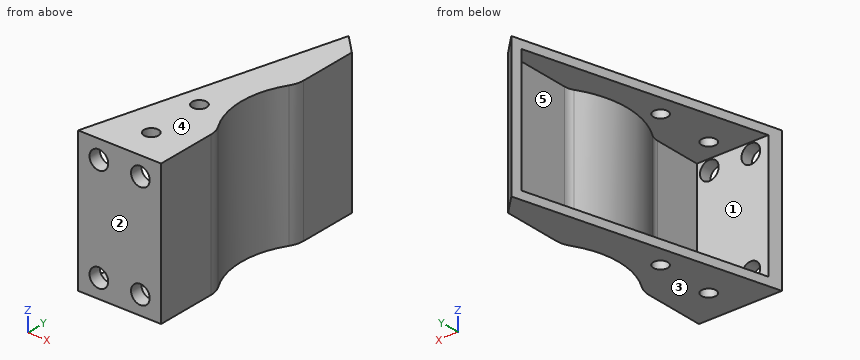
Autodesk Inventor part; units mm, degrees
ref_plane "YZ Plane" through (0, 0, 0) normal (1, 0, 0) x (0, 1, 0)
ref_plane "XZ Plane" through (0, 0, 0) normal (0, 1, 0) x (-1, 0, 0)
ref_plane "XY Plane" through (0, 0, 0) normal (0, 0, 1) x (1, 0, 0)
sketch "Sketch1" plane through (0, 0, 0) normal (0, 1, 0) x (-1, 0, 0)
  line L0 (0, 0) -> (-20, 0)
  line L1 (-20, 0) -> (-20, -34)
  line L2 (-20, -34) -> (0, -34)
  line L3 (0, -34) -> (0, 0)
  dimension "d0" = 34
  dimension "d1" = 20
extrude "Extrusion1" add sketch "Sketch1" along normal blind 60
chamfer "Chamfer1" distance 4.5 angle 45 1 edges at (20, 60, -17)
sketch "Sketch3" plane through (0, 0, 0) normal (0, 0, 1) x (1, 0, 0)
  line L0 (0, 60) -> (15.5, 60)
  line L1 (15.5, 60) -> (0, 0)
  line L2 (0, 0) -> (20, 0)
  line L3 (20, 0) -> (0, 0)
  line L4 (0, 0) -> (0, 60)
  line L5 (0, 60) -> (20, 60)
  line L6 (20, 60) -> (20, 0)
extrude "Extrusion2" cut sketch "Sketch3" against normal blind 60 contours L0 L1 L4
sketch "Sketch4" plane through (20, 0, -34) normal (0, 0, -1) x (-1, 0, 0)
  circle A0 centre (-16, 28) radius 19.8
  line L0 (0, 0) -> (0, 55.5)
  line L1 (20, 0) -> (0, 0)
  dimension "d9" = 39.6
  dimension "d14" = 16
  dimension "d15" = 28
extrude "Extrusion3" cut sketch "Sketch4" against normal blind 60
fillet "Fillet1" radius 6 2 edges at (20, 16.3364, -17) (20, 39.6636, -17)
shell "Shell1" thickness 2 removed faces 1 at (10.3333, 40, -22.6667)
sketch "Sketch5" plane through (0, 0, 0) normal (0, 0, 1) x (1, 0, 0)
  line L0 (0, 0) -> (20, 0)
  line L1 (20, 0) -> (-6.4586, 0)
  line L2 (-6.4586, 0) -> (-6.4586, 3)
  line L3 (-6.4586, 3) -> (20, 3)
  line L4 (20, 3) -> (20, 0)
  line L5 (0, 0) -> (0.775, 3)
  line L6 (15.5, 60) -> (0, 0)
  dimension "d16" = 3
extrude "Extrusion4" add sketch "Sketch5" against normal blind 34 contours L5 L3 L4 L0
sketch "Sketch6" plane through (0, 0, 0) normal (0, -1, 0) x (1, 0, 0)
  circle A0 centre (5, -4.5) radius 2.25
  line L0 (0, 0) -> (20, 0)
  line L1 (0, -34) -> (0, 0)
  circle A1 centre (15, -4.5) radius 2.25
  circle A2 centre (5, -29.5) radius 2.25
  circle A3 centre (15, -29.5) radius 2.25
  dimension "d19" = 4.5
  dimension "d20" = 4.5
  dimension "d21" = 5
  dimension "d24" = 10
  dimension "d27" = 25
extrude "Extrusion5" cut sketch "Sketch6" against normal blind 3
sketch "Sketch7" plane through (0, 0, 0) normal (0, 0, 1) x (1, 0, 0)
  circle A0 centre (11, 8) radius 1.75
  line L0 (0, 0) -> (20, 0)
  line L1 (20, 0) -> (20, 14.5226)
  line L2 (20, 0) -> (20, 15.3258)
  circle A1 centre (11, 22) radius 1.75
  dimension "d32" = 3.5
  dimension "d33" = 8
  dimension "d34" = 11
  dimension "d37" = 14
extrude "Extrusion6" cut sketch "Sketch7" against normal through all
properties part number "Gripper"
The model under review builds one solid part; all positions refer to its coordinate system, in mm. Face numbers are marked on the shaded views. A direction names the side the tool comes from. Give positions to 0.01 mm unless a question says otherwise; leave off trailing zeros. Write each loop counter-clockwise with the first axis right and the second up, starting at its lowest first coordinate (ties: lowest second). Pieces come first, ordered by that corner, then holes.
1. For P1, Ø2, axis at y = 38, z = -8, coming from the -X side; P2, Ø9, axis at y = 6.5, z = -10, coming from the -X side; P3, Ø12, axis at x = 4.5, z = -22, coming from the +Y side, all flat-tipped, find the tip position at first contact; note any pin that passes through.
2. Draft analysis for pull direction Y (two halves, no side actions). For the marked faces 1, 2 and 3, state which applies: +Y half, -Y half, draft (parallel to the pull), parting line (faces both ways), or undercut.
3. Add section A-A, the plane z = -29.5. Write out the cut boundary in (x, y) (3 decimals).
4. Add section C-C, the plane x = 5. Write out the cut boundary in (y, z).
5. Wall thickness on L1, parallel to Z at x = 5, y = 1.55; L2, parallel to Z at x = 4.5, y = 6.5; L3, parallel to X at y = 3.5, z = -25: over which ranges is each line inside the solid? List them lowest first.
6. Tool access review of the marked faces 4 and 5: name each direction out of +Z, -Z, +X, -X, +Y, -Y from which nothing blocks a thin tool from reaching the whole face with its end or side.
7. Add section D-D, the plane x = 10.5. Write out the cut boundary in (y, z).
8. Add section B-B, the plane y = 8. Write out the cut boundary in (x, z).
Worked answers:
1. P1: stops at x = 16.14
1. P2: stops at x = 0.52
1. P3: stops at y = 3
2. face 1: undercut
2. face 2: -Y half
2. face 3: draft
3. outline: (0, 0) - (2.75, 0) - (2.75, 3) - (0.775, 3) - close; (7.25, 0) - (12.75, 0) - (12.75, 3) - (7.25, 3) - close; (14.919, 57.752) - (18, 54.672) - (18, 41.477) arc R4 cw to (17.411, 39.388) arc R21.8 ccw to (17.411, 16.612) arc R4 cw to (18, 14.523) - (18, 3) - (17.25, 3) - (17.25, 0) - (20, 0) - (20, 14.523) arc R6 ccw to (19.116, 17.657) arc R19.8 cw to (19.116, 38.343) arc R6 ccw to (20, 41.477) - (20, 55.5) - (15.5, 60) - close
4. outline: (0, -34) - (19.35, -34) - (19.35, -32) - (3, -32) - (3, -31.75) - (0, -31.75) - close; (0, -27.25) - (3, -27.25) - (3, -6.75) - (0, -6.75) - close; (0, -2.25) - (3, -2.25) - (3, -2) - (19.35, -2) - (19.35, 0) - (0, 0) - close
5. L1: z = -34 to -31.75, -27.25 to -6.75, -2.25 to 0
5. L2: z = -34 to -32, -2 to 0
5. L3: x = 18 to 20
6. face 4: +Z, +X, -X, +Y, -Y
6. face 5: -X
7. outline: (0, -34) - (6.32, -34) - (6.32, -32) - (3, -32) - (3, -2) - (6.32, -2) - (6.32, 0) - (0, 0) - close; (9.68, -34) - (20.32, -34) - (20.32, -32) - (9.68, -32) - close; (9.68, -2) - (20.32, -2) - (20.32, 0) - (9.68, 0) - close; (23.68, -34) - (40.65, -34) - (40.65, -32) - (23.68, -32) - close; (23.68, -2) - (40.65, -2) - (40.65, 0) - (23.68, 0) - close
8. outline: (2.07, -34) - (9.25, -34) - (9.25, -32) - (2.07, -32) - close; (2.07, -2) - (9.25, -2) - (9.25, 0) - (2.07, 0) - close; (12.75, -34) - (20, -34) - (20, 0) - (12.75, 0) - (12.75, -2) - (18, -2) - (18, -32) - (12.75, -32) - close
